Geometry check sheet. Reference: the model listing, model coordinates, mm. A direction names the side the tool comes from. Round coordinates to 2 decimals unless told otherwise and drop trailing zeros. Loops run counter-clockwise (first coordinate to the right, second up) from the corner with the lowest first, then second, coordinate; pieces in that order, holes last. Notation, with made-up numbers: (84, 70) - (91, 70) arc R17 ccw to (91, 103) - close; hole circle Ø6 at (58.25, 6.25). An arc over 180 degrees is marked (long way). Answer as CSV lines item,"result". Start each with the question number.
1) Draft check along X on faces 4 (the flat face through (3, -3, -2)), 5 (the flat face through (79.5, -4, -1)), 6 (the flat face through (-3, -4, -1)). Enter one of: released by +X, released by -X, zero draft, split by the parting line, or undercut.
2) Cross-section at B-B on x = 76. Record the boundary of the cut face in (y, z), and give its area (3 significant figures).
3) Cross-section at A-A on y = -8.5. Record the boundary of the cut face in (x, z), and give its area (3 significant figures).
4) Depth check by flat-ended pin: P1, Ø1.5, axis at x = 10.5, y = -6, coming from the -Z side; P2, Ø1, axis at y = -7, z = -3, coming from the +X side; P3, Ø5, axis at x = 57.5, z = -7, coming from the +Y side; P4, Ø2, axis at y = 0.5, z = -6, coming from the +X side. Enter the tip coordinate at first touch or a pass-through.
5) Cross-section at D-D on x = 3. Record the boundary of the cut face in (y, z).
6) Thickness scan on line 1 along X through (y, z) = (1.25, -2.5); line 2 along X through (y, z) = (-3.5, -2.75); line 3 along Z through (x, y) = (17, 2.75). Record the ranges inside material, lowest first.
7) Cross-section at C-C on x = 62.5. Record the boundary of the cut face in (y, z).
8) Access from +Z, -Z, +X, -X, +Y, -Y to the whole of each face (thin tool, end or side, straight path). Record for faces 1 (the flat face through (70, -4, -3)), 2 (the cylindrical face through (77.526, 0.681, -6.056)), 3 (the flat face through (0, 1, -10)).
from build123d import *

# Parameters (mm, degrees)
CYLINDER_R        = 1.6
CYLINDER_DEPTH    = 10
BOX001_W          = 61
BOX001_H          = 15
BOX001_DEPTH      = 2
BOX_W             = 82.5
BOX_H             = 15
BOX_DEPTH         = 2
CYLINDER003_R     = 1.6
CYLINDER003_DEPTH = 10


with BuildPart() as taladro1:
    # Cylinder → Cylinder (new body)
    with BuildSketch(Plane(origin=(0, 1.2, -10), x_dir=(1, 0, 0), z_dir=(0, 0, 1))):
        Circle(CYLINDER_R)
    extrude(amount=CYLINDER_DEPTH)


with BuildPart() as perfora_2mm_centro:
    # Box001 → Box001 (new body)
    with BuildSketch(Plane(origin=(12, 0, -2), x_dir=(1, 0, 0), z_dir=(0, 0, 1))):
        with Locations((30.5, 7.5)):
            Rectangle(BOX001_W, BOX001_H)
    extrude(amount=BOX001_DEPTH)


with BuildPart() as fusion001:
    # Box → Box (new body)
    with BuildSketch(Plane.XY):
        with Locations((41.25, 7.5)):
            Rectangle(BOX_W, BOX_H)
    extrude(amount=BOX_DEPTH)

    # Fusion: union perfora_2mm_centro
    add(perfora_2mm_centro.part)


with BuildPart() as fusion001_1:
    # Fusion placement: moved
    add(fusion001.part.moved(Location((-3, -11, -2))))

    # Fusion001: union taladro1
    add(taladro1.part)


with BuildPart() as fusion006:
    # Cylinder003 → Cylinder003 (new body)
    with BuildSketch(Plane(origin=(76, 0.2, -10), x_dir=(1, 0, 0), z_dir=(0, 0, 1))):
        Circle(CYLINDER003_R)
    extrude(amount=CYLINDER003_DEPTH)

    # Fusion006: union Fusion001
    add(fusion001_1.part)


solid = fusion006.part
Answer block:
1,face 4,"undercut"
1,face 5,"released by +X"
1,face 6,"released by -X"
2,outline,"(-11, -2) - (-1.4, -2) - (-1.4, -10) - (1.8, -10) - (1.8, -2) - (4, -2) - (4, 0) - (-11, 0) - close"
2,area,"55.6 mm^2"
3,outline,"(-3, -2) - (9, -2) - (9, -4) - (70, -4) - (70, -2) - (79.5, -2) - (79.5, 0) - (-3, 0) - close"
3,area,"287 mm^2"
4,P1,"stops at z = -4"
4,P2,"stops at x = 70"
4,P3,"passes through"
4,P4,"stops at x = 77.6"
5,outline,"(-11, -2) - (4, -2) - (4, 0) - (-11, 0) - close"
6,line 1,"x = -1.6 to 1.6, 9 to 70, 74.79 to 77.21"
6,line 2,"x = 9 to 70"
6,line 3,"z = -4 to 0"
7,outline,"(-11, -4) - (4, -4) - (4, 0) - (-11, 0) - close"
8,face 1,"-Z, +Y, -Y"
8,face 2,"-Z"
8,face 3,"-Z, +X, -X, +Y, -Y"
